from build123d import *

# Parameters (mm, degrees)
SKETCH1_R           = 56
BOSS_EXTRUDE1_DEPTH = 4
SKETCH2_R           = 4.5
CUT_EXTRUDE1_DEPTH  = 80.296910406
SKETCH4_R           = 2
SKETCH4_R_2         = 1.5
CUT_EXTRUDE3_DEPTH  = 80.296910406


with BuildPart() as part:
    # Sketch1 → Boss-Extrude1 (new body)
    with BuildSketch(Plane(origin=(0, 0, 0), x_dir=(0, 0, -1), z_dir=(1, 0, 0))):
        Circle(SKETCH1_R)
    extrude(amount=BOSS_EXTRUDE1_DEPTH)

    # Sketch2 → Cut-Extrude1 (cut, through all)
    with BuildSketch(Plane.ZY):
        with Locations((-43.301270189, 25)):
            Circle(SKETCH2_R)
        with Locations((43.301270189, 25)):
            Circle(SKETCH2_R)
        with Locations((0, -50)):
            Circle(SKETCH2_R)
    extrude(amount=-CUT_EXTRUDE1_DEPTH, mode=Mode.SUBTRACT)

    # Sketch4 → Cut-Extrude3 (cut, through all)
    with BuildSketch(Plane(origin=(4, 0, 0), x_dir=(0, 0, -1), z_dir=(1, 0, 0))):
        with Locations((-16.75, 28.995494219)):
            Circle(SKETCH4_R)
        with Locations((16.75, 28.995494219)):
            Circle(SKETCH4_R)
        with Locations((16.75, 11)):
            Circle(SKETCH4_R)
        with Locations((-16.75, 11)):
            Circle(SKETCH4_R)
        with Locations((-37, 9)):
            Circle(SKETCH4_R_2)
        with Locations((0, -23)):
            Circle(SKETCH4_R_2)
        with Locations((37, 9)):
            Circle(SKETCH4_R_2)
    extrude(amount=-CUT_EXTRUDE3_DEPTH, mode=Mode.SUBTRACT)


solid = part.part
Read the model definition and answer for the solid it produces. Units are mm, in the model's axes. Round coordinates to 2 decimals unless told otherwise and drop trailing zeros. Write each loop counter-clockwise with the first axis right and the second up, starting at its lowest first coordinate (ties: lowest second). Pieces come first, ordered by that corner, then holes.
1. Straight lines are drawn through the part: L1, parallel to Y at x = 2.75, z = 0; L2, parallel to Z at x = 3.7, y = 29; L3, parallel to Y at x = 1.4, z = 16.75. For each, find the intervals that lie inside material, in ascending order.
2. Determine the mould class of faces 1 (the face through (1.97, -54.39, -0.98)), 2 (the face through (0, 1, 1)), 3 (the face through (1.97, -21.45, -51.73)) for opening direction Y: pulls with the +Y half, pulls with the -Y half, needs draft (parallel to the pull), parting line crosses it, or undercut.
3. The part is cut by section A-A, the plane z = 0. Determine the outline of the cut face in (x, y).
4. The part is cut by section C-C, the plane z = 37. Determine the outline of the cut face in (x, y), then the cut area to 3 significant figures.
5. The part is cut by section D-D, the plane x = 0.9. State how many separate pieces and enclosed holes the cut face has, then the cut area to 3 significant figures.
6. Given pin 1 Ø1 at (x, z) = (3.5, -29) entering from -Y; pin 2 Ø1.5 at (x, z) = (0.5, 23.5) entering from +Y; pin 3 Ø2 at (x, z) = (1, -27.5) entering from -Y; pin 4 Ø7 at (y, z) = (25, 43.3) entering from +X, each flat-ended and moving along its own axis, determine where each tip first touches the part or whether it passes through.
7. The part is cut by section B-B, the plane y = -23. Determine the outline of the cut face in (x, z).
Values:
1. L1: y = -56 to -54.5, -45.5 to -24.5, -21.5 to 56
1. L2: z = -47.91 to -45.36, -41.24 to -18.75, -14.75 to 14.75, 18.75 to 41.24, 45.36 to 47.91
1. L3: y = -53.44 to 9, 13 to 27, 31 to 53.44
2. face 1: undercut
2. face 2: needs draft
2. face 3: parting line crosses it
3. outline: (0, -56) - (4, -56) - (4, -54.5) - (0, -54.5) - close; (0, -45.5) - (4, -45.5) - (4, -24.5) - (0, -24.5) - close; (0, -21.5) - (4, -21.5) - (4, 56) - (0, 56) - close
4. outline: (0, -42.04) - (4, -42.04) - (4, 7.5) - (0, 7.5) - close; (0, 10.5) - (4, 10.5) - (4, 42.04) - (0, 42.04) - close
4. area: 324 mm2
5. separate pieces: 1
5. enclosed holes: 10
5. area: 9,590 mm2
6. pin 1: stops at y = -48.21
6. pin 2: stops at y = 51.17
6. pin 3: stops at y = -49.33
6. pin 4: passes through
7. outline: (0, -51.06) - (4, -51.06) - (4, -1.5) - (0, -1.5) - close; (0, 1.5) - (4, 1.5) - (4, 51.06) - (0, 51.06) - close
